Geometry check sheet. Reference: the model listing, model coordinates, mm. A direction names the side the tool comes from. Round coordinates to 2 decimals unless told otherwise and drop trailing zeros. Loops run counter-clockwise (first coordinate to the right, second up) from the corner with the lowest first, then second, coordinate; pieces in that order, holes last. Notation, with made-up numbers: M 22.5,-26 L 66.5,-26 A17 ccw 66.5,-12 Z; hole C 71,-36 d5. An arc over 180 degrees is marked long. Use one line per item in the form item = value. Start each with the question number.
1. Material ranges on line 1 (X direction, y = -7.5, z = 1258.5); line 2 (Z direction, x = -12.5, y = 35); line 3 (X direction, y = 23, z = 2045.5), recorded low to high.
2. Set-up check for faces 4 (the flat face through (53, -28.54, 1141)), 5 (the flat face through (3.21, 30.78, 25.01)), 6 (the flat face through (-6.655, -20, 2275)), 7 (the flat face through (3.21, -68.55, 24.32)): record each of +Z, -Z, +X, -X, +Y, -Y from which the full face is reachable in a straight line by a thin tool's end or side.
3. Cross-section at A-A (z = 1522.5). Record the boundary of the cut face in (x, y) (3 decimals), then the cut area to 3 significant figures.
4. Go/stop test with flat-tipped pins: pin 1 (16 mm diameter, centred on x = 35.5, y = -47.5, fed in from -Z); pin 2 (12 mm diameter, centred on y = 9, z = 1467.5, fed in from -X); pin 3 (10 mm diameter, centred on x = 1, z = 673.5, fed in from -Y). Record where each tip stops, or that it passes through.
5. Draft check along Y on faces 1 (the flat face through (-6.655, -68, 1141)), 2 (the flat face through (3.21, 30.78, 2224.99)), 3 (the flat face through (-46, -8.54, 1141)). Enter one of: pulls with the +Y half, pulls with the -Y half, needs draft (parallel to the pull), parting line crosses it, or undercut.
```python
from build123d import *

# Parameters (mm, degrees)
BOSS_EXTRUDE1_DEPTH = 1125
CUT_EXTRUDE1_DEPTH  = 110
BOSS_EXTRUDE2_DEPTH = 20
SKETCH4_W           = 20
SKETCH4_H           = 74.330343737
SKETCH4_H_2         = 74.330343736
BOSS_EXTRUDE3_DEPTH = 50


with BuildPart() as part:
    # Sketch1 → Boss-Extrude1 (new body)
    with BuildSketch(Plane.XY):
        with BuildLine():
            Line((77.675695624, -8.540198176), (28.345351887, -8.540198176))
            Line((28.345351887, -8.540198176), (28.345351887, -28.540198176))
            Line((28.345351887, -28.540198176), (77.675695624, -28.540198176))
            ThreePointArc((77.675695624, -28.540198176), (56.378360476, -71.573206765), (13.345351887, -92.870541913))
            Line((13.345351887, -92.870541913), (13.345351887, -43.540198176))
            Line((13.345351887, -43.540198176), (-6.654648113, -43.540198176))
            Line((-6.654648113, -43.540198176), (-6.654648113, -92.870541913))
            ThreePointArc((-6.654648113, -92.870541913), (-49.687656702, -71.573206765), (-70.984991849, -28.540198176))
            Line((-70.984991849, -28.540198176), (-21.654648113, -28.540198176))
            Line((-21.654648113, -28.540198176), (-21.654648113, -8.540198176))
            Line((-21.654648113, -8.540198176), (-70.984991849, -8.540198176))
            ThreePointArc((-70.984991849, -8.540198176), (-49.687656702, 34.492810412), (-6.654648113, 55.79014556))
            Line((-6.654648113, 55.79014556), (-6.654648113, 6.459801824))
            Line((-6.654648113, 6.459801824), (13.345351887, 6.459801824))
            Line((13.345351887, 6.459801824), (13.345351887, 55.79014556))
            ThreePointArc((13.345351887, 55.79014556), (56.378360476, 34.492810412), (77.675695624, -8.540198176))
        make_face()
    boss_extrude1 = extrude(amount=BOSS_EXTRUDE1_DEPTH)

    # Sketch2 → Cut-Extrude1 (cut, symmetric)
    with BuildSketch(Plane(origin=(0, 0, 0), x_dir=(1, 0, 0), z_dir=(0, 1, 0))):
        Polygon((-70.984991849, -140), (-38.819819981, 0), (-70.984991849, 0), align=None)
        Polygon((77.675695624, 0), (45.510523755, 0), (77.675695624, -140), align=None)
    cut_extrude1 = extrude(amount=CUT_EXTRUDE1_DEPTH, both=True, mode=Mode.SUBTRACT)

    # Sketch3 → Boss-Extrude2 (add)
    with BuildSketch(Plane(origin=(-6.654648113, 0, 0), x_dir=(0, 0, -1), z_dir=(1, 0, 0))):
        Polygon((0, 55.79014556), (0, -92.870541913), (-74.330343737, -18.540198176), align=None)
    boss_extrude2 = extrude(amount=BOSS_EXTRUDE2_DEPTH)

    # Sketch4 → Boss-Extrude3 (add)
    with BuildSketch(Plane(origin=(0, 0, 0), x_dir=(-1, 0, 0), z_dir=(0, 0, -1))):
        with Locations((-3.345351887, -55.705370045)):
            Rectangle(SKETCH4_W, SKETCH4_H)
        with Locations((-3.345351887, 18.624973692)):
            Rectangle(SKETCH4_W, SKETCH4_H_2)
    boss_extrude3 = extrude(amount=BOSS_EXTRUDE3_DEPTH)

    # Mirror1: Boss-Extrude1, Cut-Extrude1, Boss-Extrude2, Boss-Extrude3 across plane
    add(boss_extrude1.mirror(Plane.XY.offset(1125)))
    add(cut_extrude1.mirror(Plane.XY.offset(1125)), mode=Mode.SUBTRACT)
    add(boss_extrude2.mirror(Plane.XY.offset(1125)))
    add(boss_extrude3.mirror(Plane.XY.offset(1125)))


solid = part.part
```
Reported:
q1.line_1 = -70.84 to 77.53
q1.line_2 = 0 to 2250
q1.line_3 = -59.1 to -6.65, 13.35 to 65.79
q2.face_4 = +Z, -Z, +X
q2.face_5 = +Y
q2.face_6 = +Z, -X, +Y, -Y
q2.face_7 = -Y
q3.outline = M -70.985,-28.54 A75 ccw -6.655,-92.871 L -6.655,-43.54 L 13.345,-43.54 L 13.345,-92.871 A75 ccw 77.676,-28.54 L 28.345,-28.54 L 28.345,-8.54 L 77.676,-8.54 A75 ccw 13.345,55.79 L 13.345,6.46 L -6.655,6.46 L -6.655,55.79 A75 ccw -70.985,-8.54 L -21.655,-8.54 L -21.655,-28.54 Z
q3.area = 13,700 mm²
q4.pin_1 = 0
q4.pin_2 = -68.49
q4.pin_3 = -43.54
q5.face_1 = needs draft
q5.face_2 = pulls with the +Y half
q5.face_3 = undercut
